Here's how the part is built. I have some questions about the finished solid (model axes, mm). A direction names the side the tool comes from. Coordinates: 2 decimals unless noted, no trailing zeros. Order: outer loops, then holes, each group sorted by start corner. A loop starts at its lowest first (then second) coordinate and runs counter-clockwise, first axis right, second up. Notation, with made-up numbers: (-32.5, 51) - (14.5, 51) arc R18 cw to (14.5, 71) - close; hole circle Ø6 at (-1.75, -12.75). An arc over 180 degrees is marked (long way). Use CSV: the item, a comma, the result in double quotes. Start each with the question number.
from build123d import *

# Parameters (mm, degrees)
F1_DEPTH = 50.8
F3_DEPTH = 63.5
F4_W     = 50.8
F4_H     = 25.4
F5_DEPTH = 136.301493178
F6_W     = 12.6990998109
F6_H     = 38.1
F6_W_2   = 12.6558531163
F7_DEPTH = 38.1


with BuildPart() as f1:
    # F0 (on Top) → F1 (new body)
    with BuildSketch(Plane.XY):
        with BuildLine():
            Line((-177.8, 0), (0, 0))
            ThreePointArc((0, 0), (9.6159869033, 3.4237488703), (13.6063504562, 12.8187613327))
            Line((13.6063504562, 12.8187613327), (12.6990998109, 89.0133601981))
            ThreePointArc((12.6990998109, 89.0133601981), (8.9266357829, 97.8957099488), (0, 101.5621517573))
            Line((0, 101.5621517573), (-177.8, 101.5621517573))
            ThreePointArc((-177.8, 101.5621517573), (-186.7802196632, 97.842387939), (-190.4999436027, 88.8621517574))
            Line((-190.4999436027, 88.8621517574), (-190.4999436027, 12.6621517574))
            ThreePointArc((-190.4999436027, 12.6621517574), (-186.766864762, 3.7063724593), (-177.8, 0))
        make_face()
    extrude(amount=-F1_DEPTH)

    # F2 (on face) + F1_face1 (on face) → F3 (join)
    with BuildSketch(Plane.XY):
        Polygon((-38.1, 101.5621517573), (-139.7, 101.5621517573), (-88.9, 0), align=None)
    with BuildSketch(Plane(origin=(-88.6706320233, 50.7338080348, -50.8), x_dir=(1, 0, 0), z_dir=(0, 0, -1))):
        with BuildLine():
            ThreePointArc((-89.1293679767, 50.7338080348), (-98.0962327387, 47.0274355755), (-101.8293115794, 38.0716562774))
            Line((-101.8293115794, 38.0716562774), (-101.8293115794, -38.1283437226))
            ThreePointArc((-101.8293115794, -38.1283437226), (-98.1095876399, -47.1085799042), (-89.1293679767, -50.8283437225))
            Line((-89.1293679767, -50.8283437225), (88.6706320233, -50.8283437225))
            ThreePointArc((88.6706320233, -50.8283437225), (97.5972678062, -47.161901914), (101.3697318342, -38.2795521634))
            Line((101.3697318342, -38.2795521634), (102.2769824795, 37.9150467021))
            ThreePointArc((102.2769824795, 37.9150467021), (98.2866189266, 47.3100591645), (88.6706320233, 50.7338080348))
            Line((88.6706320233, 50.7338080348), (-89.1293679767, 50.7338080348))
        make_face()
    extrude(amount=F3_DEPTH, dir=(0, 0, 1))

    # F4 (on face) → F5 (cut, through all)
    with BuildSketch(Plane(origin=(-71.109398148, 35.5679489201, 0), x_dir=(0.4473469078, 0.8943605224, 0), z_dir=(0.8943605224, -0.4473469078, 0))):
        with Locations((-14.3691401044, 37.928833447)):
            Rectangle(F4_W, F4_H)
    extrude(amount=-F5_DEPTH, mode=Mode.SUBTRACT)

    # F6 (on face) → F7 (cut)
    with BuildSketch(Plane(origin=(13.7570332765, 0.1638052763, 0), x_dir=(-0.0119061764, 0.999929119, 0), z_dir=(0.999929119, 0.0119061764, 0))):
        with Locations((95.2054030218, -31.75)):
            Rectangle(F6_W, F6_H)
        with Locations((6.3279265582, -31.75)):
            Rectangle(F6_W_2, F6_H)
        Polygon((64.6785830399, 12.7), (37.2213781047, 12.7), (37.2213781047, -12.7), (12.6558531163, -12.7), (12.6558531163, -50.8), (88.8558531163, -50.8), (88.8558531163, -12.7), (64.6785830399, -12.7), align=None)
    extrude(amount=-F7_DEPTH, mode=Mode.SUBTRACT)


solid = f1.part
Item 1: Suppose I cut it at B-B on x = -17. Write out the boundary of the cut face in (y, z), then the cut area to 3 significant figures.
Item 2: Suppose I cut it at D-D on z = 3. Write out the boundary of the cut face in (x, y).
Item 3: For pin 1 Ø8 at (x, z) = (-114, 29.5) entering from -Y; pin 2 Ø1.5 at (x, z) = (-167, -18.5) entering from -Y; pin 3 Ø8 at (x, y) = (-45.5, 30.5) entering from +Z, each with a flat end and sliding along its axis, tell me the tip position at first contact or that it passes through.
Item 4: Suppose I cut it at C-C on y = 10. Write out the boundary of the cut face in (x, z).
Item 5: For faces 1 (the flat face through (-152, 50, 12.7)), 2 (the flat face through (-96.1, 60.4, 37.8)), 3 (the flat face through (-58.211, 61.355, 37.744)), which set-ups out of +Z, -Z, +X, -X, +Y, -Y let a thin tool reach every point of the face, with its end or its side?
Item 6: Suppose I cut it at A-A on z = -18. Write out the boundary of the cut face in (x, y), then the cut area to 3 significant figures.
Item 7: Please list where these lines run through material, in increasing order: line 1 along Z through (x, y) = (-90, 41); line 2 along Z through (x, y) = (-123.5, 42); line 3 along X through (y, z) = (14, -1.5). Write a range as from..to.
Here are the results:
1,outline,"(0, -12.7) - (37.02, -12.7) - (37.02, 12.7) - (0, 12.7) - close; (64.48, -12.7) - (101.36, -12.7) - (101.36, -50.8) - (101.56, -50.8) - (101.56, 12.7) - (64.48, 12.7) - close"
1,area,"1,890 mm^2"
2,outline,"(-190.5, 12.66) arc R12.7 ccw to (-177.8, 0) - (0, 0) arc R12.7 ccw to (13.61, 12.82) - (13.31, 37.38) - (-24.78, 36.93) - (-25.11, 64.38) - (12.99, 64.84) - (12.7, 89.01) arc R12.7 ccw to (0, 101.56) - (-177.8, 101.56) arc R12.7 ccw to (-190.5, 88.86) - close"
3,pin 1,"y = 67.35"
3,pin 2,"y = 0"
3,pin 3,"z = 12.7"
4,outline,"(-190.21, -50.8) - (-24.46, -50.8) - (-24.46, -12.7) - (13.32, -12.7) - (13.32, 12.7) - (-83.9, 12.7) - (-83.9, 25.23) - (-93.9, 25.23) - (-93.9, 12.7) - (-190.21, 12.7) - close; (-93.9, 50.63) - (-83.9, 50.63) - (-83.9, 63.5) - (-93.9, 63.5) - close"
5,face 1,"+Z, -X, -Y"
5,face 2,"-X, -Y"
5,face 3,"+Z, +X, -Y"
6,outline,"(-190.5, 12.66) arc R12.7 ccw to (-177.8, 0) - (-24.34, 0) - (-25.55, 101.26) - (0, 101.56) - (-177.8, 101.56) arc R12.7 ccw to (-190.5, 88.86) - close; (0, 0) arc R12.7 ccw to (2.12, 0.03) - close"
6,area,"16,700 mm^2"
7,line 1,"-50.8..25.23, 50.63..63.5"
7,line 2,"-50.8..12.7"
7,line 3,"-190.5..13.59"
